The model under review builds one solid part; all positions refer to its coordinate system, in mm. Face numbers are marked on the shaded views. A direction names the side the tool comes from. Round coordinates to 2 decimals unless told otherwise and drop trailing zeros. Write each loop counter-clockwise with the first axis right and the second up, starting at its lowest first coordinate (ties: lowest second). Pieces come first, ordered by that corner, then holes. Notation, with made-up numbers: (-6.5, -22) - (39.5, -22) arc R20 ccw to (39.5, -14) - close; hole circle Ø9 at (-35.5, -15). An arc over 180 degrees is marked (long way). Write each question's results on one line, items separated by ' | '.
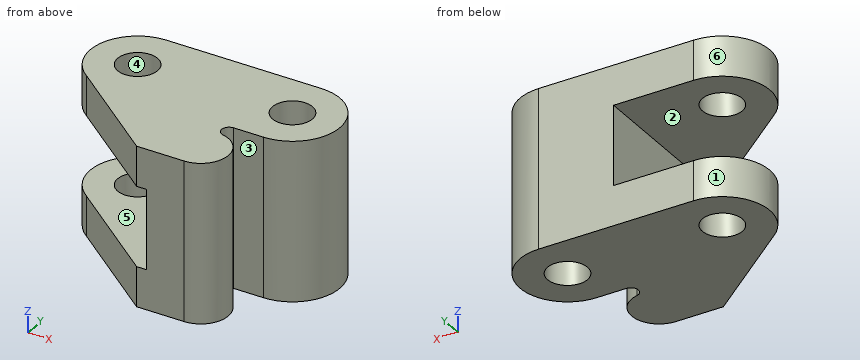
Autodesk Inventor part; units mm, degrees
ref_plane "YZ Plane" through (0, 0, 0) normal (1, 0, 0) x (0, 1, 0)
ref_plane "XZ Plane" through (0, 0, 0) normal (0, 1, 0) x (-1, 0, 0)
sketch "Sketch1" plane through (0, 0, 0) normal (0, 0, 1) x (1, 0, 0)
  circle A0 centre (31, -9.5) radius 4 construction
  circle A1 centre (0, -9.5) radius 4 construction
  line L0 (31, 0) -> (0, 0)
  arc A2 (0, 0) -> (-5.5818, -17.1873) centre (0, -9.5) ccw
  line L1 (14, -32.8402) -> (-5.5818, -17.1873)
  line L2 (23.513, -32.8402) -> (14, -32.8402)
  arc A3 (23.513, -32.8402) -> (24.6813, -21.9658) centre (23.513, -27.3402) ccw
  arc A4 (25, -19) -> (24.6813, -21.9658) centre (25, -20.5) ccw
  line L3 (31, -19) -> (25, -19)
  arc A5 (31, -19) -> (31, 0) centre (31, -9.5) ccw
  point P0 (0, 0)
  dimension "d0" = 9.5
  dimension "d1" = 8
  dimension "d2" = 31
  dimension "d3" = 1.5
  dimension "d4" = 5.5
  dimension "d6" = 9.513
  dimension "d7" = 38.638
  dimension "d9" = 32.8402
  dimension "d10" = 16.9104
extrude "Extrusion1" add sketch "Sketch1" along normal mid plane 32
sketch "Sketch2" plane through (14, -32.8402, 16) normal (0, -1, 0) x (1, 0, 0)
  line L0 (0, -32) -> (0, 0)
  line L1 (-23.5, -32) -> (-23.5, 0)
  line L2 (-23.5, -24) -> (2, -24)
  line L3 (2, -24) -> (2, -8)
  line L4 (2, -8) -> (-23.5, -8)
  line L5 (-23.5, -8) -> (-23.5, -24)
  point P0 (-23.5, -16)
  dimension "d13" = 2
  dimension "d14" = 16
extrude "Extrusion2" cut sketch "Sketch2" against normal through all
hole "Hole1" at (31, -9.5, 16) direction (0, 0, -1) diameter 8 end through all
hole "Hole2" at (0, -9.5, 16) direction (0, 0, -1) diameter 8 end through all
equation "\"LENGTH\" = 25.4"
properties part number "TU-008"
Q1. We need section B-B (z = 14). State the section outline as (x, y) points, plus the area to 3 significant figures.
Evaluation:
outline: (-5.58, -17.19) - (14, -32.84) - (23.51, -32.84) arc R5.5 ccw to (24.68, -21.97) arc R1.5 cw to (25, -19) - (31, -19) arc R9.5 ccw to (31, 0) - (0, 0) arc R9.5 ccw to start; hole circle Ø8 at (0, -9.5); hole circle Ø8 at (31, -9.5) | area: 1,070 mm^2
Q2. The part is to be moulded in two halves that separate along X. For the marked faces 4, 5 and 6, say which applies: released by +X, released by -X, zero draft, split by the parting line, or undercut.
Evaluation:
face 4: undercut | face 5: zero draft | face 6: released by -X
Q3. We need section D-D (y = -2). State the section outline as (x, z) points.
Evaluation:
outline: (-5.83, -16) - (36.83, -16) - (36.83, 16) - (-5.83, 16) - (-5.83, 8) - (16, 8) - (16, -8) - (-5.83, -8) - close
Q4. We need section C-C (z = 7). State the section outline as (x, y) points, plus the area to 3 significant figures.
Evaluation:
outline: (16, -32.84) - (23.51, -32.84) arc R5.5 ccw to (24.68, -21.97) arc R1.5 cw to (25, -19) - (31, -19) arc R9.5 ccw to (31, 0) - (16, 0) - close; hole circle Ø8 at (31, -9.5) | area: 529 mm^2
Q5. For probe 1 along X at (y, z) = (-9.5, 11); probe 2 along Z at (x, y) = (-1, -3.5); probe 3 along X at (y, z) = (-9.5, 7.5), list the stretches that pass through material, from the lowest coordinate up.
Evaluation:
probe 1: x = -9.5 to -4, 4 to 27, 35 to 40.5 | probe 2: z = -16 to -8, 8 to 16 | probe 3: x = 16 to 27, 35 to 40.5
Q6. Insertion check: P1, Ø5, axis at y = -6, z = 6, coming from the -X side; P2, Ø6.5, axis at x = 0, y = -9.5, coming from the -Z side; P3, Ø17.5, axis at y = -18, z = 1, coming from the -X side; P4, Ø1.8, axis at x = 26.5, z = 2.5, coming from the -Y side. Each pin has a flat end and moves straight along its axis. Give the tip position at first contact, or say it passes through.
Evaluation:
P1: stops at x = -9.29 | P2: passes through | P3: stops at x = -8.93 | P4: stops at y = -32.43
Q7. Tool access review of the marked faces 1, 2 and 3: name each direction out of +Z, -Z, +X, -X, +Y, -Y from which nothing blocks a thin tool from reaching the whole face with its end or side.
Evaluation:
face 1: +Z, -Z, -X | face 2: -X, +Y, -Y | face 3: +Z, -Z, +X
Q8. We need section A-A (x = 7). State the section outline as (y, z) points.
Evaluation:
outline: (-27.24, -16) - (0, -16) - (0, -8) - (-27.24, -8) - close; (-27.24, 8) - (0, 8) - (0, 16) - (-27.24, 16) - close
